Can you work these out from the drawing? Everything is in mm from the part's minimum corner. A direction names the side the tool comes from. Round coordinates to 2 decimals unless told otherwise and drop trailing zeros. Loops run counter-clockwise (first coordinate to the right, second up) from the corner with the lowest first, then second, coordinate; pieces in that order, holes last. Notation, with made-up numbers: M 31.5,-31 L 41.5,-31 A23 ccw 41.5,-15 Z; hole C -37.5,43 d5. An arc over 180 degrees is marked long. One line per question, with ' | ' between items. Start each with the question number.
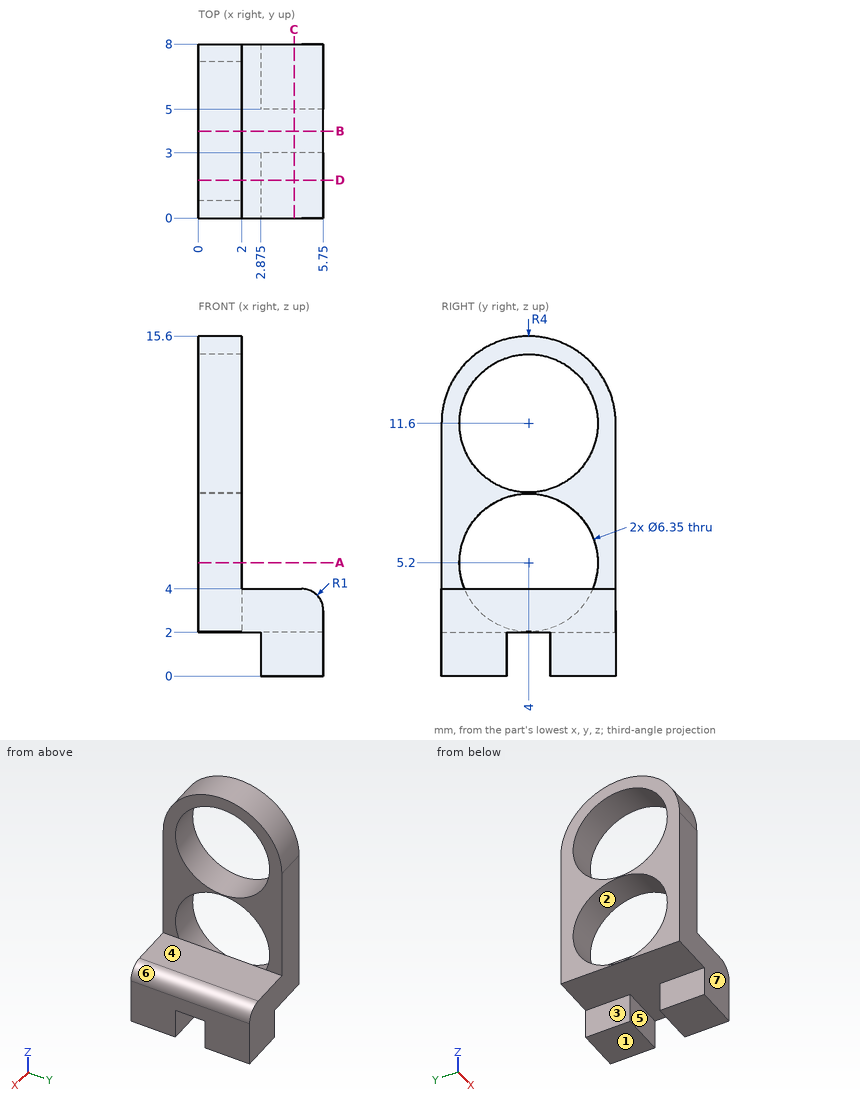
1) Please list where these lines run through material, in increasing order: L1, parallel to Y at x = 1, z = 5.2 (3 decimals); L2, parallel to Z at x = 1.85, y = 6.75; L3, parallel to Y at x = 0.3, z = 6.5. Write a range as from..to.
2) For the marked faces 1, 2, 3 and 4, which set-ups out of +Z, -Z, +X, -X, +Y, -Y let a thin tool reach every point of the face, with its end or its side?
3) We'd pull the mould along Y, two halves only. Please class the marked faces 5, 6 and 7: pulls with the +Y half, pulls with the -Y half, needs draft (parallel to the pull), parting line crosses it, or undercut.
4) Imagine slicing it at B-B (y = 4). Write out the boundary of the cut face in (x, z) (3 decimals), then the cut area to 3 significant figures.
5) Imagine slicing it at A-A (z = 5.2). Write out the boundary of the cut face in (x, y) (3 decimals).
6) Imagine slicing it at C-C (x = 4.4). Write out the boundary of the cut face in (y, z), then the cut area to 3 significant figures.
7) I'm going to push flat-ended pins straight in: pin 1 Ø1 at (x, z) = (5, 1.5) entering from -Y; pin 2 Ø1.6 at (y, z) = (1, 0.5) entering from -X (3 decimals); pin 3 Ø4 at (y, z) = (2, 12) entering from +X; pin 4 Ø1.4 at (x, y) = (3.5, 2.5) entering from +Z. Where does each tip first touch, or does it pass through?
8) Imagine slicing it at D-D (y = 1.75). Write out the boundary of the cut face in (x, z) (3 decimals), then the cut area to 3 significant figures.
Results are:
1) L1: 0..0.825, 7.175..8 | L2: 2..3.61, 6.79..10.01, 13.19..14.5 | L3: 0..1.1, 6.9..8
2) face 1: -Z, +X, -X, +Y, -Y | face 2: -X | face 3: -Z, -X, +Y, -Y | face 4: +Z, +X, +Y, -Y
3) face 5: undercut | face 6: needs draft | face 7: pulls with the -Y half
4) outline: M 0,2 L 5.75,2 L 5.75,3 A1 ccw 4.75,4 L 2,4 L 2,2.025 L 0,2.025 Z; M 0,8.375 L 2,8.375 L 2,8.425 L 0,8.425 Z; M 0,14.775 L 2,14.775 L 2,15.6 L 0,15.6 Z | area: 9.09 mm²
5) outline: M 0,0 L 2,0 L 2,0.825 L 0,0.825 Z; M 0,7.175 L 2,7.175 L 2,8 L 0,8 Z
6) outline: M 0,0 L 3,0 L 3,2 L 5,2 L 5,0 L 8,0 L 8,4 L 0,4 Z | area: 28.0 mm²
7) pin 1: y = 0 | pin 2: x = 2.875 | pin 3: x = 2 | pin 4: z = 4
8) outline: M 0,2 L 2.875,2 L 2.875,0 L 5.75,0 L 5.75,3 A1 ccw 4.75,4 L 2,4 L 2,2.96 L 0,2.96 Z; M 0,7.44 L 2,7.44 L 2,9.36 L 0,9.36 Z; M 0,13.84 L 2,13.84 L 2,14.907 L 0,14.907 Z | area: 20.9 mm²
